Autodesk Inventor part; units mm, degrees
ref_plane "YZ Plane" through (0, 0, 0) normal (1, 0, 0) x (0, 1, 0)
ref_plane "XZ Plane" through (0, 0, 0) normal (0, 1, 0) x (-1, 0, 0)
ref_plane "XY Plane" through (0, 0, 0) normal (0, 0, 1) x (1, 0, 0)
sketch "Sketch1" plane through (0, 0, 0) normal (0, 1, 0) x (-1, 0, 0)
  line L0 (15, 14.965) -> (-15, 14.965)
  line L1 (-15, 14.965) -> (-15, -14.965)
  line L2 (-15, -14.965) -> (15, -14.965)
  line L3 (15, -14.965) -> (15, 14.965)
  point P0 (0, 0)
  dimension "d0" = 29.93
  dimension "d1" = 30
  dimension "d2" = 15
  dimension "d3" = 14.965
extrude "Plate1" add sketch "Sketch1" along normal blind 1.5
sketch "Sketch2" plane through (-15, 0, -13.465) normal (0, 0, -1) x (-1, 0, 0)
  line L0 (-30, 0) -> (0, 0)
  line L1 (0, 0) -> (0, 43)
  line L2 (0, 43) -> (-30, 43)
  line L3 (-30, 43) -> (-30, 0)
edge flange "Flange1" height 43 angle 90 thickness 1.5 bend radius 0.31 thickness toward (0, 0, -1) relief tear relief width 1.5 relief depth 0.75 corner gap 0.31 corner form 0 edges at (0, 1.5, -14.965) (0, 1.5, 14.965) wall of the first edge with corners at (15, 0, -13.465) (-15, 0, -13.465) (-15, 43, -13.465) (15, 43, -13.465)
bend "Bend1"
corner "Corner1"
sketch "Sketch3" plane through (-15, 43, 14.965) normal (0, 0, 1) x (1, 0, 0)
  line L0 (0, 0) -> (30, 0)
  line L1 (0, -41.19) -> (0, 0)
  circle A0 centre (15, -10) radius 10
  line L2 (0, -18.5) -> (30, -18.5)
  line L3 (30, -18.5) -> (30, -28.5)
  line L4 (30, -28.5) -> (0, -28.5)
  line L5 (0, -28.5) -> (0, -18.5)
  line L6 (30, -18.5) -> (24.0624, -5.7723)
  line L7 (0, -18.5) -> (5.9376, -5.7723)
  line L8 (0, 0) -> (30, 0)
  line L9 (30, 0) -> (30, -25)
  line L10 (30, -25) -> (0, -25)
  line L11 (0, -25) -> (0, 0)
  point P0 (15, -43)
  point P1 (15, 0)
  dimension "d15" = 10
  dimension "d16" = 0
  dimension "d17" = 20
  dimension "d18" = 8.5
  dimension "d19" = 0
  dimension "d20" = 30
  dimension "d21" = 10
  dimension "d22" = 25
extrude "Extrusion1" cut sketch "Sketch3" against normal blind 35 contours L0 A0 L7 L1 | L0 L9 L6 A0
sketch "Sketch4" plane through (15, 1.81, -14.965) normal (0, 0, -1) x (-1, 0, 0)
  arc A0 (24.0624, 35.4177) -> (5.9376, 35.4177) centre (15, 31.19) ccw
  circle A1 centre (15, 31.19) radius 2.6
  circle A2 centre (8, 31.19) radius 1.05
  circle A3 centre (22, 31.19) radius 1.05
  circle A4 centre (15, 38.19) radius 1.05
  circle A5 centre (15, 24.19) radius 1.05
  point P0 (15, -1.81)
  dimension "d25" = 5.2
  dimension "d26" = 0
  dimension "d27" = 7
  dimension "d28" = 2.1
  dimension "d29" = 7
  dimension "d30" = 0
  dimension "d31" = 2.1
  dimension "d32" = 0
  dimension "d33" = 7
  dimension "d34" = 2.1
  dimension "d35" = 7
  dimension "d36" = 0
  dimension "d37" = 2.1
extrude "Extrusion2" cut sketch "Sketch4" against normal blind 1.5
sketch "Sketch5" plane through (-15, 1.81, 14.965) normal (0, 0, 1) x (1, 0, 0)
  arc A0 (24.0624, 35.4177) -> (5.9376, 35.4177) centre (15, 31.19) ccw
  circle A1 centre (15, 31.19) radius 2.55
  point P0 (15, -1.81)
  dimension "d40" = 5.1
extrude "Extrusion3" cut sketch "Sketch5" against normal blind 1.5
sketch "Sketch6" plane through (0, 1.5, 0) normal (0, 1, 0) x (1, 0, 0)
  circle A0 centre (-7, 1.535) radius 0.7835
  circle A1 centre (0, 8.535) radius 0.7835
  circle A2 centre (7, 1.535) radius 0.7835
  circle A3 centre (0, -5.465) radius 0.7835
  circle A4 centre (0, 1.535) radius 1.75
  circle A5 centre (0, 1.535) radius 9.96
  point P0 (0, 0)
hole "Hole1" at (-7, 1.5, -1.535) at (0, 1.5, 5.465) at (7, 1.5, -1.535) at (0, 1.5, -8.535) direction (0, -1, 0) diameter 2.1 depth 1.5
sketch "Sketch7" plane through (0, 1.5, 0) normal (0, 1, 0) x (1, 0, 0)
  circle A0 centre (0, 1.535) radius 1.75
  point P0 (0, 0)
hole "Hole2" at (0, 1.5, -1.535) direction (0, -1, 0) diameter 5.2 depth 1.5
equation "\"d48\" = Thickness"
equation "\"d55\" = Thickness"
equation "\"d4\" = Thickness"
equation "\"d5\" = BendReliefWidth"
equation "\"d6\" = BendReliefDepth"
equation "\"d7\" = MinimumRemnant"
equation "\"d8\" = TransitionRadius"
equation "\"d11\" = BendRadius"
equation "\"d12\" = CornerReliefSize"
equation "\"d13\" = GapSize"
equation "\"d14\" = JacobiRadiusSize"
equation "\"BendReliefWidth\" = Thickness"
equation "\"BendReliefDepth\" = 0.5 * Thickness"
equation "\"CornerReliefSize\" = 4 * Thickness"
equation "\"MinimumRemnant\" = 2 * Thickness"
equation "\"TransitionRadius\" = BendRadius"
equation "\"JacobiRadiusSize\" = BendRadius"
equation "\"GapSize\" = Thickness"
properties part number "partpart" material "Aluminum 6061-AHC"
Verification items for the finished model (mm, model axes). A direction names the side the tool comes from. Give positions to 0.01 mm unless a question says otherwise; leave off trailing zeros. Write each loop counter-clockwise with the first axis right and the second up, starting at its lowest first coordinate (ties: lowest second). Pieces come first, ordered by that corner, then holes. Notation, with made-up numbers: M -1,58.5 L 48,58.5 A6 ccw 48,64.5 Z; hole C 61,-7.5 d4. An arc over 180 degrees is marked long. Write item = value, one per line.
(1) Sectioned sample at C-C (x = 0). Give the number of separate pieces and of enclosed holes in the cut face, then the cut area to 3 significant figures.
Found:
separate_pieces = 8
enclosed_holes = 0
area = 132 mm2
(2) Sectioned sample at B-B (y = 33). Record the cut outline in (x, z) (3 decimals).
Found:
outline = M -11.035,-14.965 L -8.05,-14.965 L -8.05,-13.465 L -11.035,-13.465 Z; M -11.035,13.465 L -2.55,13.465 L -2.55,14.965 L -11.035,14.965 Z; M -5.95,-14.965 L -2.6,-14.965 L -2.6,-13.465 L -5.95,-13.465 Z; M 2.55,13.465 L 11.035,13.465 L 11.035,14.965 L 2.55,14.965 Z; M 2.6,-14.965 L 5.95,-14.965 L 5.95,-13.465 L 2.6,-13.465 Z; M 8.05,-14.965 L 11.035,-14.965 L 11.035,-13.465 L 8.05,-13.465 Z
(3) Sectioned sample at D-D (z = -8). Record the cut outline in (x, y), then the cut area to 3 significant figures.
Found:
outline = M -15,0 L -0.9,0 L -0.9,1.5 L -15,1.5 Z; M 0.9,0 L 15,0 L 15,1.5 L 0.9,1.5 Z
area = 42.3 mm2
(4) Material ranges on line 1 (Z direction, x = 9, y = 26.5) (3 decimals); line 2 (Y direction, x = 5, z = 5.5); line 3 (Y direction, x = 7, z = -14.5), recorded low to high.
Found:
line_1 = -14.965 to -13.465, 13.465 to 14.965
line_2 = 0 to 1.5
line_3 = 0.6 to 31.95, 34.05 to 40.14
(5) Access from +Z, -Z, +X, -X, +Y, -Y to the whole of each face (thin tool, end or side, straight path). Record for faces 4 (the face through (0, 18, 13.465)), 5 (the face through (-6.772, 31.975, -14.226)), 6 (the face through (-7.315, 0.74, -0.533)).
Found:
face_4 = +X, -X, +Y
face_5 = -Z
face_6 = +Y, -Y
(6) Draft check along Z on faces 1 (the face through (-0.33, 35.53, 14.23)), 2 (the face through (0, 18, -14.965)), 3 (the face through (-0.046, 0.74, 4.416)). Enter one of: released by +Z, released by -Z, zero draft, split by the parting line, or undercut.
Found:
face_1 = zero draft
face_2 = released by -Z
face_3 = undercut
(7) Sectioned sample at A-A (y = 11). Record the cut outline in (x, z) (3 decimals).
Found:
outline = M -15,-14.965 L 15,-14.965 L 15,-13.465 L -15,-13.465 Z; M -15,13.465 L 15,13.465 L 15,14.965 L -15,14.965 Z
(8) Go/stop test with flat-tipped pins: pin 1 Ø4.5 at (x, z) = (0, -1.535) entering from +Y; pin 2 Ø1.3 at (x, y) = (-7, 33) entering from -Z (3 decimals); pin 3 Ø10 at (x, z) = (-6, -9) entering from +Y; pin 4 Ø3.5 at (x, z) = (-7, -1.535) entering from +Y. Record where each tip stops, or that it passes through.
Found:
pin_1 = through
pin_2 = 13.465
pin_3 = 42.27
pin_4 = 1.5
